Autodesk Inventor part; units mm, degrees
ref_plane "YZ Plane" through (0, 0, 0) normal (1, 0, 0) x (0, 1, 0)
ref_plane "XZ Plane" through (0, 0, 0) normal (0, 1, 0) x (-1, 0, 0)
ref_plane "XY Plane" through (0, 0, 0) normal (0, 0, 1) x (1, 0, 0)
ref_plane "Work Plane1" through (0, 0, 0) normal (0, 0, 1) x (1, 0, 0)
sketch "Sketch1" plane through (0, 0, 0) normal (0, 0, 1) x (1, 0, 0)
  line L0 (12.6235, -7.6637) -> (25.0692, -36.6156)
  arc A0 (25.2873, -37.408) -> (25.0692, -36.6156) centre (22.3131, -37.8003) ccw
  line L1 (25.2873, -37.408) -> (29.8752, -72.1865)
  arc A1 (28.1539, -74.4309) -> (29.8752, -72.1865) centre (27.8924, -72.448) ccw
  line L2 (28.1539, -74.4309) -> (7.7764, -77.119)
  arc A2 (7.7764, -77.119) -> (8.9535, -86.0417) centre (8.365, -81.5803) ccw
  line L3 (8.9535, -86.0417) -> (37.2623, -82.3073)
  arc A3 (37.2623, -82.3073) -> (39.8442, -78.9407) centre (36.8699, -79.3331) ccw
  line L4 (39.8442, -78.9407) -> (34.0473, -34.997)
  arc A4 (34.0473, -34.997) -> (33.8292, -34.2046) centre (31.073, -35.3894) ccw
  line L5 (33.8292, -34.2046) -> (20.8924, -4.1103)
  arc A5 (20.4398, -2.6174) -> (20.8924, -4.1103) centre (27.3234, -1.3458) ccw
  line L6 (20.4398, -2.6174) -> (14.5173, 29.4432)
  arc A6 (14.405, 30.9564) -> (14.5173, 29.4432) centre (21.4008, 30.7148) ccw
  line L7 (14.405, 30.9564) -> (15.7585, 70.1518)
  arc A7 (15.7585, 70.1518) -> (13.7755, 73.0784) centre (12.7603, 70.2554) ccw
  line L8 (13.7755, 73.0784) -> (-21.8863, 85.9033)
  arc A8 (-21.8863, 85.9033) -> (-25.7246, 84.0956) centre (-22.9016, 83.0803) ccw
  line L9 (-25.7246, 84.0956) -> (-39.6044, 45.5005)
  arc A9 (-39.6044, 45.5005) -> (-31.1354, 42.4548) centre (-35.3699, 43.9777) ccw
  line L10 (-31.1354, 42.4548) -> (-28.9682, 48.481)
  arc A10 (-23.2109, 51.1927) -> (-28.9682, 48.481) centre (-24.7337, 46.9582) ccw
  line L11 (-23.2109, 51.1927) -> (2.9943, 41.7686)
  arc A11 (5.6382, 37.8666) -> (2.9943, 41.7686) centre (1.6406, 38.0046) ccw
  line L12 (5.6382, 37.8666) -> (5.4104, 31.2681)
  arc A12 (5.4104, 31.2681) -> (5.5231, 29.7528) centre (12.4062, 31.0266) ccw
  line L13 (5.5231, 29.7528) -> (12.1714, -6.1729)
  arc A13 (12.1714, -6.1729) -> (12.6235, -7.6637) centre (19.0545, -4.8992) ccw
  circle A14 centre (29.5855, -35.7988) radius 1.55
  circle A15 centre (10.5349, 68.7475) radius 1.55
  circle A16 centre (16.4901, -5.1537) radius 1.55
  circle A17 centre (-21.4682, 80.037) radius 1.55
  circle A18 centre (-35.3699, 43.9777) radius 1.55
  circle A19 centre (34.3649, -77.4119) radius 1.55
  circle A20 centre (-28.5644, 59.2229) radius 1.55
  circle A21 centre (8.365, -81.5803) radius 1.55
  circle A22 centre (9.9227, 30.3521) radius 1.55
  line L14 (0.9032, 52.0849) -> (-20.6357, 59.8309)
  arc A23 (-23.0461, 64.9485) -> (-20.6357, 59.8309) centre (-19.2821, 63.5949) ccw
  line L15 (-23.0461, 64.9485) -> (-20.3013, 72.5809)
  arc A24 (-16.463, 74.3887) -> (-20.3013, 72.5809) centre (-17.4783, 71.5657) ccw
  line L16 (-16.463, 74.3887) -> (3.8682, 67.077)
  arc A25 (6.5122, 63.1749) -> (3.8682, 67.077) centre (2.5146, 63.313) ccw
  line L17 (6.5122, 63.1749) -> (6.2544, 55.7109)
  arc A26 (0.9032, 52.0849) -> (6.2544, 55.7109) centre (2.2568, 55.8489) ccw
  line L18 (-14.3316, 28.4241) -> (-19.7537, 49.0626) construction
  line L19 (1.5801, -32.1414) -> (-3.5777, -12.5091) construction
  line L20 (-6.8942, 0.1146) -> (-11.0151, 15.8005) construction
  line L21 (-25.7315, 60.0097) -> (-31.5346, 58.4851) construction
  line L22 (-19.8838, 37.7512) -> (-25.7315, 60.0097) construction
  line L23 (-25.6869, 36.2266) -> (-19.8838, 37.7512) construction
  line L24 (-25.6869, 36.2266) -> (-31.5346, 58.4851) construction
  line L25 (1.5128, -67.305) -> (7.3158, -65.7804) construction
  line L26 (10.8632, -102.8959) -> (1.5128, -67.305) construction
  line L27 (16.6662, -101.3713) -> (10.8632, -102.8959) construction
  line L28 (7.3158, -65.7804) -> (16.6662, -101.3713) construction
  line L29 (-20.011, 50.0419) -> (13.2082, -76.4024)
  arc A27 (-27.5927, 78.9008) -> (-20.011, 50.0419) centre (8.9141, 73.0664) ccw
  point P0 (0, 0)
extrude "Extrusion1" add sketch "Sketch1" along normal blind 1 contours A13 L13 A12 L12 A11 L11 A27 L9 A8 L8 A7 L7 A6 L6 A5 L5 A4 L4 A3 L3 A2 L2 A1 L1 A0 L0 | L0 A0 L1 A1 L2 L29 L11 A11 L12 A12 L13 A13 | L14 A23 L15 A24 L16 A25 L17 A26
properties part number "side skert v2" material "Brass, Soft Yellow"
The listing builds one solid part. Answer for the finished solid, in the listing's coordinates (mm). A direction names the side the tool comes from. Round coordinates to 2 decimals unless told otherwise and drop trailing zeros. Order: outer loops, then holes, each group sorted by start corner. A loop starts at its lowest first (then second) coordinate and runs counter-clockwise, first axis right, second up. Notation, with made-up numbers: M 35.5,61 L 43.5,61 A13 ccw 43.5,85 Z; hole C -19,82 d4. An arc over 180 degrees is marked long. Answer in a Markdown table with one row per item. Add a question column.
1) The part is cut by section A-A on z = 0.5. Count the separate pieces of the cut face and the enclosed holes in it, plus the area to 3 significant figures.
2) A flat-ended cylindrical pin translates along its axis: pin 1 Ø3 at (x, y) = (0.5, -38.5) entering from -Z. Find the tip coordinate at first contact, or state that the pin passes through.
3) Determine the mould class of faces 4 (the face through (5, 1, 1)), 5 (the face through (36.986, -57.276, 0.493)), 6 (the face through (5, 1, 0)) for opening direction Z: pulls with the +Z half, pulls with the -Z half, needs draft (parallel to the pull), parting line crosses it, or undercut.
4) Which of the six approach directions +Z, -Z, +X, -X, +Y, -Y give full straight-line access (tool end or side, diameter ignored) to faces 1 (the face through (17.52, 13.19, 0.49)), 2 (the face through (-3.634, -12.295, 0.493)), 3 (the face through (10.638, 31.727, 0.493))?
5) The part is cut by section C-C on y = -22. Determine the outline of the cut face in (x, z).
6) Consider line 1 along Y through (x, z) = (22.5, 0.85); line 2 along X through (y, z) = (-18.5, 0.2); line 3 along X through (y, z) = (60, 0.15). Determine where each line is inside the solid, lowest interval first. Write a range as from..to.
7) The part is cut by section B-B on x = -4. Determine the outline of the cut face in (y, z), plus the area to 3 significant figures.
Findings below:
| question | item | result |
|---|---|---|
| 1 | separate pieces | 1 |
| 1 | enclosed holes | 7 |
| 1 | area | 5,150 mm² |
| 2 | pin 1 | passes through |
| 3 | face 4 | pulls with the +Z half |
| 3 | face 5 | needs draft |
| 3 | face 6 | pulls with the -Z half |
| 4 | face 1 | +Z, -Z, +X |
| 4 | face 2 | +Z, -Z, -X |
| 4 | face 3 | +Z, -Z |
| 5 | outline | M -1.08,0 L 28.58,0 L 28.58,1 L -1.08,1 Z |
| 6 | line 1 | y = -84.25..-7.85 |
| 6 | line 2 | x = -2..27.08 |
| 6 | line 3 | x = -25.67..15.41 |
| 7 | outline | M -10.9,0 L 79.47,0 L 79.47,1 L -10.9,1 Z |
| 7 | area | 90.4 mm² |
